Read the model definition and answer for the solid it produces. Units are mm, in the model's axes. A direction names the side the tool comes from. Give positions to 0.01 mm unless a question says otherwise; leave off trailing zeros. Order: outer loops, then holes, each group sorted by start corner. A loop starts at its lowest first (then second) coordinate and runs counter-clockwise, first axis right, second up. Notation, with made-up numbers: M 18,24 L 77,24 A24 cw 77,37 Z; hole C -13,-26 d8. An arc over 180 degrees is marked long. One line per item, written item: value. Start each with the question number.
from build123d import *

# Parameters (mm, degrees)
SKETCH4_R                        = 7.9375
EXTRUDE1_DEPTH                   = 101.6
F_11_32_0_34375_DIAMETER_HOLE1_D = 8.73252


with BuildPart() as part:
    # Sketch1 → Revolve1 (revolve)
    with BuildSketch(Plane.XY):
        Polygon((0, 0), (20.32, 0), (20.32, -7.62), (15.706148476, -7.62), (15.706148476, -9.525), (0, -9.525), align=None)
    revolve(axis=Axis((158.75, 0, 0), (1, 0, 0)))

    # Sketch4 → Extrude1 (add)
    with BuildSketch(Plane(origin=(20.32, 0, 0), x_dir=(0, 0, -1), z_dir=(1, 0, 0))):
        Circle(SKETCH4_R)
    extrude(amount=EXTRUDE1_DEPTH)

    # Sketch5 → Revolve2 (revolve)
    with BuildSketch(Plane.XY):
        Polygon((121.92, 6.35), (132.354619201, 6.35), (132.354619201, 4.733622738), (138.281335828, 4.733622738), (138.281335828, 6.35), (142.322278983, 6.35), (142.322278983, 0), (121.92, 0), align=None)
    revolve(axis=Axis((142.322278983, 0, 0), (-1, 0, 0)))

    # 11/32 (0.34375) Diameter Hole1 (through all)
    with Locations(Plane(origin=(7.108304199, 2.913032452, 9.068619902), x_dir=(0, 0.952086079, -0.305830179), z_dir=(0, 0.305830179, 0.952086079))):
        with Locations((0, 0)):
            Hole(F_11_32_0_34375_DIAMETER_HOLE1_D / 2)


solid = part.part
Q1. Determine the mould class of faces 4 (the flat face through (121.92, 7, 0)), 5 (the cylindrical face through (11.37, 0.86, -0.42)), 6 (the cylindrical face through (70.41, -7.75, 1.72)) for opening direction Y: released by +Y, released by -Y, zero draft, split by the parting line, or undercut.
Q2. Find section A-A, the plane x = 73. Give the vertices of the cut face in (y, z) (1 decimal), then the cut area to 3 significant figures.
Q3. Consider probe 1 along Z at (x, y) = (108.5, 4.75); probe 2 along X at (y, z) = (1.75, -3.5); probe 3 along Y at (x, z) = (123.5, -0.5). Determine where each line is inside the solid, lowest interval first.
Q4. A tool of negligible diameter and unlimited length cuts with its end or side. For faces 1 (the cylindrical face through (140.33, -1.38, 6.2)), 2 (the cylindrical face through (7.743, 7.559, 5.796)), 3 (the flat face through (132.355, -5, 0)), from which of +Z, -Z, +X, -X, +Y, -Y can it reach the whole face along a straight path? Write none if from no direction.
Q5. Each of these flat-tipped pins is pushed along its axis until it touches: pin 1 (2 mm diameter, centred on x = 125.5, z = -1.5, fed in from +Y); pin 2 (1.5 mm diameter, centred on x = 91, z = 2, fed in from -Y); pin 3 (6 mm diameter, centred on x = 58.5, z = -3, fed in from +Y); pin 4 (4 mm diameter, centred on y = 0.5, z = -3, fed in from -X). Where does it stop, or does it pass through?
Evaluation:
1. face 4: zero draft
1. face 5: undercut
1. face 6: split by the parting line
2. outline: C 0,0 d15.9
2. area: 198 mm2
3. probe 1: -6.36 to 6.36
3. probe 2: 0 to 3.71, 10.51 to 142.32
3. probe 3: -6.33 to 6.33
4. face 1: +X
4. face 2: +X, -X
4. face 3: none
5. pin 1: y = 6.33
5. pin 2: y = -7.84
5. pin 3: y = 7.94
5. pin 4: x = 0
